Verification items for the finished model (mm, model axes). Face numbers are marked on the shaded views. A direction names the side the tool comes from. Coordinates: 2 decimals unless noted, no trailing zeros. Write each loop counter-clockwise with the first axis right and the second up, starting at its lowest first coordinate (ties: lowest second). Pieces come first, ordered by that corner, then holes. Notation, with made-up numbers: M 84.5,-29.5 L 120.5,-29.5 A16 ccw 120.5,-13.5 Z; hole C 3,54.5 d10. An arc over 180 degrees is marked long. One line per item, written item: value.
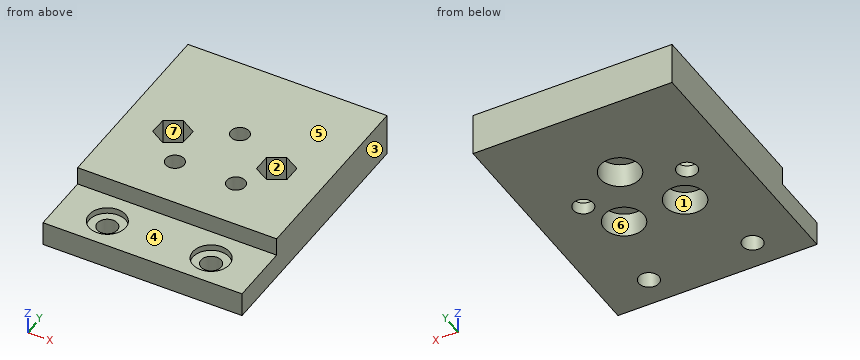
```python
from build123d import *

# Parameters (mm, degrees)
SKICA1_W                 = 32.614180818
SKICA1_H                 = 41.995577694
SKICA1_R                 = 1.649999753
SKICA1_R_2               = 1.649999979
SKICA1_R_3               = 1.649999826
SKICA1_R_4               = 1.650000122
P_IDAT_VYSUNUT_M1_DEPTH  = 4
ODEBRAT_VYSUNUT_M1_DEPTH = 3
SKICA3_W                 = 32.614180818
SKICA3_H                 = 31.955890059
P_IDAT_VYSUNUT_M2_DEPTH  = 3
SKICA4_R                 = 1.649999753
SKICA4_R_2               = 1.649999979
P_IDAT_VYSUNUT_M3_DEPTH  = 1
SKICA5_R                 = 3
ODEBRAT_VYSUNUT_M2_DEPTH = 1
SKICA6_R                 = 1.5
SKICA6_R_2               = 1.495454726
ODEBRAT_VYSUNUT_M3_DEPTH = 7
SKICA7_R                 = 3.25
ODEBRAT_VYSUNUT_M4_DEPTH = 4


with BuildPart() as part:
    # Skica1 → Přidat vysunutím1 (new body)
    with BuildSketch(Plane.XY):
        with Locations((0, 6.659801208)):
            Rectangle(SKICA1_W, SKICA1_H)
        with Locations((-8.49999961, 9.500000046)):
            Circle(SKICA1_R, mode=Mode.SUBTRACT)
        with Locations((8.499999866, 9.50000039)):
            Circle(SKICA1_R_2, mode=Mode.SUBTRACT)
        with Locations((8.500000308, -9.499999987)):
            Circle(SKICA1_R_3, mode=Mode.SUBTRACT)
        with Locations((-8.499999537, -9.500000426)):
            Circle(SKICA1_R_4, mode=Mode.SUBTRACT)
    extrude(amount=P_IDAT_VYSUNUT_M1_DEPTH)

    # Skica2 → Odebrat vysunutím1 (cut)
    with BuildSketch(Plane.XY.offset(4)):
        Polygon((-8.437315747, 12.386070743), (-10.968068219, 10.997321212), (-11.030752082, 8.111250516), (-8.562683473, 6.61392935), (-6.031931001, 8.002678881), (-5.969247138, 10.888749577), align=None)
        Polygon((8.499999866, 12.386751736), (5.999999866, 10.943376063), (5.999999866, 8.056624717), (8.499999866, 6.613249044), (10.999999866, 8.056624717), (10.999999866, 10.943376063), align=None)
    extrude(amount=-ODEBRAT_VYSUNUT_M1_DEPTH, mode=Mode.SUBTRACT)

    # Skica3 → Přidat vysunutím2 (add)
    with BuildSketch(Plane.XY.offset(4)):
        with Locations((0, 11.679645025)):
            Rectangle(SKICA3_W, SKICA3_H)
        Polygon((-8.437315747, 12.386070743), (-10.968068219, 10.997321212), (-11.030752082, 8.111250516), (-8.562683473, 6.61392935), (-6.031931001, 8.002678881), (-5.969247138, 10.888749577), align=None, mode=Mode.SUBTRACT)
        Polygon((10.999999866, 10.943376063), (8.499999866, 12.386751736), (5.999999866, 10.943376063), (5.999999866, 8.056624717), (8.499999866, 6.613249044), (10.999999866, 8.056624717), align=None, mode=Mode.SUBTRACT)
    extrude(amount=P_IDAT_VYSUNUT_M2_DEPTH)

    # Skica4 → Přidat vysunutím3 (add)
    # profile 1 of 2: a face of its own
    with BuildSketch(Plane.XY.offset(1)):
        Polygon((-5.969247138, 10.888749577), (-8.437315747, 12.386070743), (-10.968068219, 10.997321212), (-11.030752082, 8.111250516), (-8.562683473, 6.61392935), (-6.031931001, 8.002678881), align=None)
        with Locations((-8.49999961, 9.500000046)):
            Circle(SKICA4_R, mode=Mode.SUBTRACT)
    # profile 2 of 2: a face of its own
    with BuildSketch(Plane.XY.offset(1)):
        Polygon((10.999999866, 10.943376063), (8.499999866, 12.386751736), (5.999999866, 10.943376063), (5.999999866, 8.056624717), (8.499999866, 6.613249044), (10.999999866, 8.056624717), align=None)
        with Locations((8.499999866, 9.50000039)):
            Circle(SKICA4_R_2, mode=Mode.SUBTRACT)
    extrude(amount=P_IDAT_VYSUNUT_M3_DEPTH)

    # Skica5 → Odebrat vysunutím2 (cut)
    with BuildSketch(Plane.XY.offset(4)):
        with Locations((8.500000308, -9.499999987)):
            Circle(SKICA5_R)
        with Locations((-8.499999537, -9.500000426)):
            Circle(SKICA5_R)
    extrude(amount=-ODEBRAT_VYSUNUT_M2_DEPTH, mode=Mode.SUBTRACT)

    # Skica6 → Odebrat vysunutím3 (cut)
    with BuildSketch(Plane.XY.offset(7)):
        with Locations((5.107090409, 3.701699996)):
            Circle(SKICA6_R)
        with Locations((-4.892909591, 3.701699996)):
            Circle(SKICA6_R)
        with Locations((0.107090409, 13.701699996)):
            Circle(SKICA6_R_2)
    extrude(amount=-ODEBRAT_VYSUNUT_M3_DEPTH, mode=Mode.SUBTRACT)

    # Skica7 → Odebrat vysunutím4 (cut)
    with BuildSketch(Plane(origin=(0, 0, 0), x_dir=(-1, 0, 0), z_dir=(0, 0, -1))):
        with Locations((4.892909591, 3.701699996)):
            Circle(SKICA7_R)
        with Locations((-5.107090409, 3.701699996)):
            Circle(SKICA7_R)
        with Locations((-0.107090409, 13.701699996)):
            Circle(SKICA7_R)
    extrude(amount=-ODEBRAT_VYSUNUT_M4_DEPTH, mode=Mode.SUBTRACT)


solid = part.part
```
Item 1: Cross-section at B-B, the plane x = 7.5. Enter the section's corners in (y, z).
The answers:
outline: M -14.34,0 L -10.81,0 L -10.81,3 L -12.33,3 L -12.33,4 L -14.34,4 Z; M -8.19,0 L 1.5,0 L 1.5,4 L 5.9,4 L 5.9,0 L 8.19,0 L 8.19,2 L 7.19,2 L 7.19,7 L -4.3,7 L -4.3,4 L -6.67,4 L -6.67,3 L -8.19,3 Z; M 10.81,0 L 27.66,0 L 27.66,7 L 11.81,7 L 11.81,2 L 10.81,2 Z
Item 2: Cross-section at A-A, the plane y = -9.5. Enter the section's corners in (x, z).
The answers:
outline: M -16.31,0 L -10.15,0 L -10.15,3 L -11.5,3 L -11.5,4 L -16.31,4 Z; M -6.85,0 L 6.85,0 L 6.85,3 L 5.5,3 L 5.5,4 L -5.5,4 L -5.5,3 L -6.85,3 Z; M 10.15,0 L 16.31,0 L 16.31,4 L 11.5,4 L 11.5,3 L 10.15,3 Z
Item 3: Draft check along X on the marked faces 1, 2, 3 and 4. Enter one of: released by +X, released by -X, zero draft, split by the parting line, or undercut.
The answers:
face 1: undercut
face 2: undercut
face 3: released by +X
face 4: zero draft
Item 4: Access from +Z, -Z, +X, -X, +Y, -Y to the whole of each face (thin tool, end or side, straight path). Record for the marked faces 5, 6 and 7.
The answers:
face 5: +Z, +X, -X, +Y, -Y
face 6: -Z
face 7: +Z
Item 5: Cross-section at D-D, the plane z = 5.25. Enter the section's corners in (x, y), and give its area (3 significant figures).
The answers:
outline: M -16.31,-4.3 L 16.31,-4.3 L 16.31,27.66 L -16.31,27.66 Z; hole M -11.03,8.11 L -8.56,6.61 L -6.03,8 L -5.97,10.89 L -8.44,12.39 L -10.97,11 Z; hole C -4.89,3.7 d3; hole C 0.11,13.7 d2.99; hole C 5.11,3.7 d3; hole M 6,8.06 L 8.5,6.61 L 11,8.06 L 11,10.94 L 8.5,12.39 L 6,10.94 Z
area: 978 mm²
Item 6: Cross-section at C-C, the plane x = -5. Enter the section's corners in (y, z).
The answers:
outline: M -14.34,0 L 0.45,0 L 0.45,4 L 2.21,4 L 2.21,7 L -4.3,7 L -4.3,4 L -14.34,4 Z; M 5.2,4 L 6.95,4 L 6.95,0 L 27.66,0 L 27.66,7 L 5.2,7 Z
Item 7: Scan lines: line 1 (X direction, y = 8.5, z = 6.25); line 2 (Y direction, x = 2.5, z = 3); line 3 (X direction, y = 1.5, z = 2.5). Record each from-to range of solid material in increasing order.
The answers:
line 1: x = -16.31 to -11.02, -6.02 to 6, 11 to 16.31
line 2: y = -14.34 to 1.76, 5.64 to 11.5, 15.9 to 27.66
line 3: x = -16.31 to -7.28, -2.5 to 2.72, 7.5 to 16.31
Item 8: Go/stop test with flat-tipped pins: P1, Ø3.5, axis at x = -4.89, y = 3.7, coming from the -Z side; P2, Ø2.5, axis at x = -8.5, y = 9.5, coming from the +Z side; P3, Ø2, axis at x = 6.5, z = 5.5, coming from the -Y side; P4, Ø1.5, axis at x = -9.5, y = 10.5, coming from the +Z side. Record where each tip stops, or that it passes through.
The answers:
P1: stops at z = 4
P2: passes through
P3: stops at y = -4.3
P4: stops at z = 2
